Input: part model. Units: mm. Frame: model coordinates. Face numbers are marked on the shaded views. A direction names the side the tool comes from. Coordinates: 2 decimals unless noted, no trailing zeros. Write each loop counter-clockwise with the first axis right and the second up, starting at its lowest first coordinate (ties: lowest second). Pieces come first, ordered by that corner, then holes. Notation, with made-up numbers: M 8,43.25 L 50,43.25 A16 cw 50,54.25 Z; hole C 60.25,67.25 d6. An arc over 180 degrees is marked long. Write each question's results on one line, items separated by ' | '. Start each with the question number.
1. First-contact query: pin 1 (8 mm diameter, centred on y = 9, z = -86.5, fed in from -X); pin 2 (12 mm diameter, centred on x = -70, z = 0, fed in from -Y); pin 3 (4 mm diameter, centred on x = 35.5, z = -68, fed in from -Y); pin 4 (12 mm diameter, centred on x = 31.5, y = 9.5, fed in from -Z). Flat tips, straight axial feed; report the tip coordinate or a pass-through.
2. Section query C-C, the plane x = 0. Output: boundary loops of the cut face in (y, z).
3. Set-up query: the marked faces 5, 6 and 7. Return all of +Z, -Z, +X, -X, +Y, -Y with unobstructed straight access to the full face (end or side cutting, diameter ignored); none if empty.
4. Ray query, probe 1 along X at (y, z) = (14.5, -88); probe 2 along Z at (x, y) = (57, 20); probe 3 along Z at (x, y) = (64.5, 23.5). Return the intervals inside material, ascending.
5. Section query D-D, the plane x = -24. Output: boundary loops of the cut face in (y, z), and give its area (3 significant figures).
6. Pull-direction query (X, two-part tool) for the marked faces 1, 2, 3 and 4; classes: +X half, -X half, draft (parallel to the pull), parting line (faces both ways), or undercut.
7. Section query A-A, the plane z = -88. Output: boundary loops of the cut face in (x, y).
8. Section query B-B, the plane y = 27. Output: boundary loops of the cut face in (x, z), and give its area (3 significant figures).
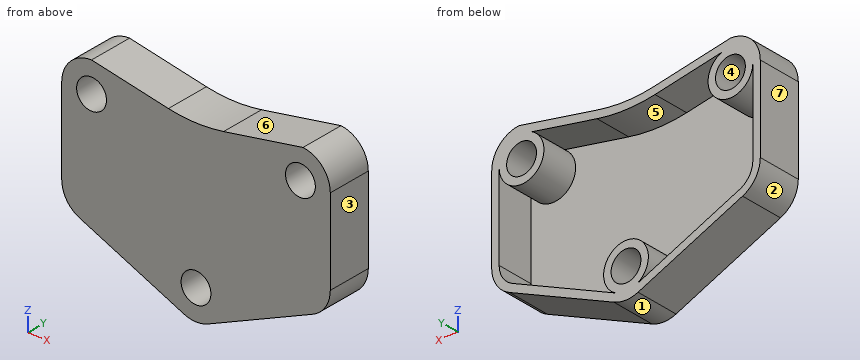
```python
from build123d import *

# Parameters (mm, degrees)
SKETCH1_R           = 10
BOSS_EXTRUDE1_DEPTH = 30
SHELL3_START        = 5
SHELL3_DEPTH        = 25


# Read off the part's stored shape, not the designer's step: Shell3
with BuildPart() as part:
    # Sketch1 → Boss-Extrude1 (new body)
    with BuildSketch(Plane(origin=(0, 0, 0), x_dir=(1, 0, 0), z_dir=(0, 1, 0))):
        with BuildLine():
            Line((90, 0), (90, 57.047137228))
            ThreePointArc((90, 57.047137228), (86.75954181, 67.961245451), (78.088224169, 75.338682537))
            Line((78.088224169, 75.338682537), (8.088224169, 106.291545309))
            ThreePointArc((8.088224169, 106.291545309), (0, 108), (-8.088224169, 106.291545309))
            Line((-8.088224169, 106.291545309), (-78.088224169, 75.338682537))
            ThreePointArc((-78.088224169, 75.338682537), (-86.75954181, 67.961245451), (-90, 57.047137228))
            Line((-90, 57.047137228), (-90, 0))
            ThreePointArc((-90, 0), (-84.142135624, -14.142135624), (-70, -20))
            Line((-70, -20), (-18.49195659, -10.161261295))
            ThreePointArc((-18.49195659, -10.161261295), (0.004664589, -8.385754022), (18.510453887, -10.063008789))
            Line((18.510453887, -10.063008789), (71.68950902, -19.928511216))
            ThreePointArc((71.68950902, -19.928511216), (84.727358561, -13.531626281), (90, 0))
        make_face()
        with Locations(Location((-70, 0, 0), (0, 0, 270))):
            Circle(SKETCH1_R, mode=Mode.SUBTRACT)
        with Locations(Location((70, 0, 0), (0, 0, 270))):
            Circle(SKETCH1_R, mode=Mode.SUBTRACT)
        with Locations(Location((0, 88, 0), (0, 0, 270))):
            Circle(SKETCH1_R, mode=Mode.SUBTRACT)
    extrude(amount=BOSS_EXTRUDE1_DEPTH)

    # Shell3 outline → Shell3 (cut)
    with BuildSketch(Plane(origin=(0, 0, 0), x_dir=(1, 0, 0), z_dir=(0, 1, 0)).offset(SHELL3_START)):
        with BuildLine():
            Line((-85, 57.047137228), (-85, 0))
            ThreePointArc((-85, 0), (-61.754503332, 12.530434338), (-64.065095374, -13.775953944))
            Line((-64.065095374, -13.775953944), (-19.430064103, -5.250054285))
            ThreePointArc((-19.430064103, -5.250054285), (-0.008611865, -3.385771649), (19.422466898, -5.146889154))
            Line((19.422466898, -5.146889154), (62.898194489, -13.212280594))
            ThreePointArc((62.898194489, -13.212280594), (62.303477495, 12.874919081), (85, 0))
            Line((85, 0), (85, 57.047137228))
            ThreePointArc((85, 57.047137228), (82.569656358, 65.232718395), (76.066168127, 70.765796209))
            Line((76.066168127, 70.765796209), (6.066168127, 101.718658982))
            ThreePointArc((6.066168127, 101.718658982), (0, 73), (-6.066168127, 101.718658982))
            Line((-6.066168127, 101.718658982), (-76.066168127, 70.765796209))
            ThreePointArc((-76.066168127, 70.765796209), (-82.569656358, 65.232718395), (-85, 57.047137228))
        make_face()
    extrude(amount=SHELL3_DEPTH, mode=Mode.SUBTRACT)


solid = part.part
```
Answer:
1) pin 1: x = -61.89 | pin 2: through | pin 3: y = 0 | pin 4: z = -98.59
2) outline: M 0,-108 L 30,-108 L 30,-98 L 0,-98 Z; M 0,-78 L 30,-78 L 30,-73 L 5,-73 L 5,3.39 L 30,3.39 L 30,8.39 L 0,8.39 Z
3) face 5: +Y | face 6: +Z, +Y, -Y | face 7: +Z, -Z, -X, +Y, -Y
4) probe 1: -49.45 to -37.09, -15 to -10, 10 to 15, 37.09 to 49.45 | probe 2: -84.66 to -79.2, -7.48 to 7.48, 12.12 to 17.2 | probe 3: -81.35 to -75.88, -13.96 to -8.35, 8.35 to 18.59
5) outline: M 0,-99.26 L 30,-99.26 L 30,-93.79 L 5,-93.79 L 5,6.12 L 30,6.12 L 30,11.21 L 0,11.21 Z | area: 816 mm^2
6) face 1: parting line | face 2: -X half | face 3: +X half | face 4: undercut
7) outline: M -49.45,0 L -10,0 L -10,30 L -15,30 L -15,5 L -37.09,5 L -37.09,30 L -49.45,30 Z; M 10,0 L 49.45,0 L 49.45,30 L 37.09,30 L 37.09,5 L 15,5 L 15,30 L 10,30 Z
8) outline: M -90,-57.05 A20 ccw -78.09,-75.34 L -8.09,-106.29 A20 ccw 8.09,-106.29 L 78.09,-75.34 A20 ccw 90,-57.05 L 90,0 A20 ccw 71.69,19.93 L 18.51,10.06 A100 cw -18.49,10.16 L -70,20 A20 ccw -90,0 Z; hole M -85,-57.05 A15 ccw -76.07,-70.77 L -6.07,-101.72 A15 cw long 6.07,-101.72 L 76.07,-70.77 A15 ccw 85,-57.05 L 85,0 A15 cw long 62.9,13.21 L 19.42,5.15 A105 cw -19.43,5.25 L -64.07,13.78 A15 cw long -85,0 Z; hole C -70,0 d20; hole C 0,-88 d20; hole C 70,0 d20 | area: 3,770 mm^2
